```python
from build123d import *

# Parameters (mm, degrees)
SKETCH1_W           = 745
SKETCH1_H           = 825
SKETCH1_W_2         = 140
SKETCH1_H_2         = 665
SKETCH1_W_3         = 105
BOSS_EXTRUDE1_DEPTH = 200


with BuildPart() as part:
    # Sketch1 → Boss-Extrude1 (new body)
    with BuildSketch(Plane(origin=(0, 0, 0), x_dir=(1, 0, 0), z_dir=(0, 1, 0))):
        Rectangle(SKETCH1_W, SKETCH1_H)
        with Locations((-222.5, 0)):
            Rectangle(SKETCH1_W_2, SKETCH1_H_2, mode=Mode.SUBTRACT)
        with Locations((222.5, 0)):
            Rectangle(SKETCH1_W_2, SKETCH1_H_2, mode=Mode.SUBTRACT)
        Rectangle(SKETCH1_W_3, SKETCH1_H_2, mode=Mode.SUBTRACT)
    extrude(amount=BOSS_EXTRUDE1_DEPTH)


solid = part.part
```
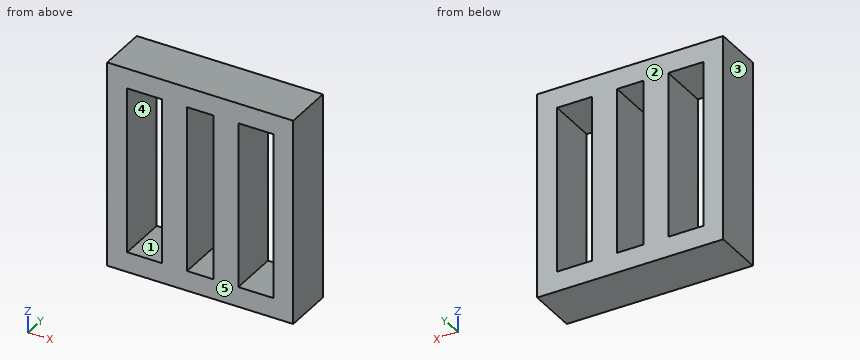
Geometry check sheet. Reference: the model listing, model coordinates, mm. Face numbers are marked on the shaded views. A direction names the side the tool comes from. Coordinates: 2 decimals unless noted, no trailing zeros. Order: outer loops, then holes, each group sorted by start corner. A loop starts at its lowest first (then second) coordinate and runs counter-clockwise, first axis right, second up. Notation, with made-up numbers: (81.25, 21.25) - (85.25, 21.25) arc R25 cw to (85.25, 47.25) - close; hole circle Ø5 at (-3, 87.25). An arc over 180 degrees is marked (long way). Answer as a JSON object with one key per item and string values. Group by question number.
Item 1: Draft check along X on the marked faces 1, 2 and 3. Enter one of: +X half, -X half, draft (parallel to the pull), parting line (faces both ways), or undercut.
Item 2: Sectioned sample at B-B, the plane y = 41. Record the cut outline in (x, z).
Item 3: Sectioned sample at A-A, the plane x = -263.5. Record the cut outline in (y, z), and give its area (3 significant figures).
Item 4: Sectioned sample at C-C, the plane z = 87. Record the cut outline in (x, y).
Item 5: Scan lines: probe 1 along X at (y, z) = (170, 162.5); probe 2 along Z at (x, y) = (249, 156). Record each from-to range of solid material in increasing order.
Item 6: Tool access check on the marked faces 4 and 5. Record the directions out of +Z, -Z, +X, -X, +Y, -Y that give a thin tool (end or side, any length) a straight path to the whole face; none if there is none.
Resolved:
{
 "1": {"face 1": "undercut", "face 2": "draft", "face 3": "-X half"},
 "2": {"outline": "(-372.5, -412.5) - (372.5, -412.5) - (372.5, 412.5) - (-372.5, 412.5) - close; hole (-292.5, -332.5) - (-152.5, -332.5) - (-152.5, 332.5) - (-292.5, 332.5) - close; hole (-52.5, -332.5) - (52.5, -332.5) - (52.5, 332.5) - (-52.5, 332.5) - close; hole (152.5, -332.5) - (292.5, -332.5) - (292.5, 332.5) - (152.5, 332.5) - close"},
 "3": {"outline": "(0, -412.5) - (200, -412.5) - (200, -332.5) - (0, -332.5) - close; (0, 332.5) - (200, 332.5) - (200, 412.5) - (0, 412.5) - close", "area": "32,000 mm^2"},
 "4": {"outline": "(-372.5, 0) - (-292.5, 0) - (-292.5, 200) - (-372.5, 200) - close; (-152.5, 0) - (-52.5, 0) - (-52.5, 200) - (-152.5, 200) - close; (52.5, 0) - (152.5, 0) - (152.5, 200) - (52.5, 200) - close; (292.5, 0) - (372.5, 0) - (372.5, 200) - (292.5, 200) - close"},
 "5": {"probe 1": "-372.5 to -292.5, -152.5 to -52.5, 52.5 to 152.5, 292.5 to 372.5", "probe 2": "-412.5 to -332.5, 332.5 to 412.5"},
 "6": {"face 4": "+Y, -Y", "face 5": "+Z, -Z, +X, -X, -Y"}
}
